The model under review builds one solid part; all positions refer to its coordinate system, in mm. Face numbers are marked on the shaded views. A direction names the side the tool comes from. Give positions to 0.01 mm unless a question says otherwise; leave off trailing zeros. Order: outer loops, then holes, each group sorted by start corner. A loop starts at its lowest first (then second) coordinate and runs counter-clockwise, first axis right, second up. Notation, with made-up numbers: (4, -10) - (22, -10) arc R30 ccw to (22, 25) - close; hole circle Ø1 at (0, 89.25). An arc over 180 degrees is marked (long way). Answer as CSV lines item,"result". Start each with the question number.
from build123d import *

# Parameters (mm, degrees)
SKETCH_1_R          = 18.5
EXTRUDE_1_DEPTH     = 7
EXTRUDE_2_DEPTH     = 4
SKETCH_2_R          = 17.5
CUT_EXTRUDE_1_DEPTH = 3
SKETCH_3_R          = 14
CUT_EXTRUDE_2_DEPTH = 2
CUT_EXTRUDE_5_REACH = 34.299
SKETCH_8_R          = 5.1
CUT_EXTRUDE_6_REACH = 34.16
SKETCH_11_R         = 1.5
FILLET_1_R          = 10
FILLET_2_R          = 5
SKETCH_12_W         = 3
SKETCH_12_H         = 2.288293169
CUT_EXTRUDE_7_DEPTH = 3


with BuildPart() as part:
    # 草图1 → 凸台-拉伸1 (new body)
    with BuildSketch(Plane(origin=(0, 0, 0), x_dir=(0, 0, -1), z_dir=(1, 0, 0))):
        Circle(SKETCH_1_R)
    extrude(amount=EXTRUDE_1_DEPTH)

    # 草图10 → 凸台-拉伸2 (add)
    with BuildSketch(Plane.ZY):
        Polygon((0, 5), (26, 5), (26, -5), (0, -5), (-26, -5), (-26, 5), align=None)
    extrude(amount=-EXTRUDE_2_DEPTH)

    # 草图2 → 切除-拉伸1 (cut)
    with BuildSketch(Plane(origin=(7, 0, 0), x_dir=(0, 0, -1), z_dir=(1, 0, 0))):
        Circle(SKETCH_2_R)
    extrude(amount=-CUT_EXTRUDE_1_DEPTH, mode=Mode.SUBTRACT)

    # 草图3 → 切除-拉伸2 (cut)
    with BuildSketch(Plane(origin=(4, 0, 0), x_dir=(0, 0, -1), z_dir=(1, 0, 0))):
        Circle(SKETCH_3_R)
    extrude(amount=-CUT_EXTRUDE_2_DEPTH, mode=Mode.SUBTRACT)

    # 草图8 → 切除-拉伸5 (cut, up to next)
    with BuildSketch(Plane(origin=(2, 0, 0), x_dir=(0, 0, -1), z_dir=(1, 0, 0)), mode=Mode.PRIVATE) as cut_extrude_5_sk1:
        Circle(SKETCH_8_R)
    cut_extrude_5_tool1 = extrude(cut_extrude_5_sk1.sketch, amount=-CUT_EXTRUDE_5_REACH, mode=Mode.PRIVATE) & part.part
    add(cut_extrude_5_tool1.solids().sort_by_distance((2, 0, 0))[0], mode=Mode.SUBTRACT)

    # 草图11 → 切除-拉伸6 (cut, up to next)
    with BuildSketch(Plane(origin=(4, 0, 0), x_dir=(0, 0, -1), z_dir=(1, 0, 0)), mode=Mode.PRIVATE) as cut_extrude_6_sk1:
        with Locations((-22, 0)):
            Circle(SKETCH_11_R)
    cut_extrude_6_tool1 = extrude(cut_extrude_6_sk1.sketch, amount=-CUT_EXTRUDE_6_REACH, mode=Mode.PRIVATE) & part.part
    # 草图11 → 切除-拉伸6 (cut, up to next)
    with BuildSketch(Plane(origin=(4, 0, 0), x_dir=(0, 0, -1), z_dir=(1, 0, 0)), mode=Mode.PRIVATE) as cut_extrude_6_sk2:
        with Locations((22, 0)):
            Circle(SKETCH_11_R)
    cut_extrude_6_tool2 = extrude(cut_extrude_6_sk2.sketch, amount=-CUT_EXTRUDE_6_REACH, mode=Mode.PRIVATE) & part.part
    add(cut_extrude_6_tool1.solids().sort_by_distance((4, 0, 22))[0], mode=Mode.SUBTRACT)
    add(cut_extrude_6_tool2.solids().sort_by_distance((4, 0, -22))[0], mode=Mode.SUBTRACT)

    # 圆角1
    fillet_1_edges = [part.edges().sort_by_distance(p)[0] for p in [
        (2, 5, -17.811513131),
        (2, 5, 17.811513131),
        (2, -5, 17.811513131),
        (2, -5, -17.811513131),
    ]]
    fillet(fillet_1_edges, radius=FILLET_1_R)

    # 圆角2
    fillet_2_edges = [part.edges().sort_by_distance(p)[0] for p in [
        (2, 5, 26),
        (2, -5, 26),
        (2, -5, -26),
        (2, 5, -26),
    ]]
    fillet(fillet_2_edges, radius=FILLET_2_R)

    # 草图12 → 切除-拉伸7 (cut)
    with BuildSketch(Plane(origin=(7, 0, 0), x_dir=(0, 0, -1), z_dir=(1, 0, 0))):
        with Locations((0, 18.044159171)):
            Rectangle(SKETCH_12_W, SKETCH_12_H)
    extrude(amount=-CUT_EXTRUDE_7_DEPTH, mode=Mode.SUBTRACT)


solid = part.part
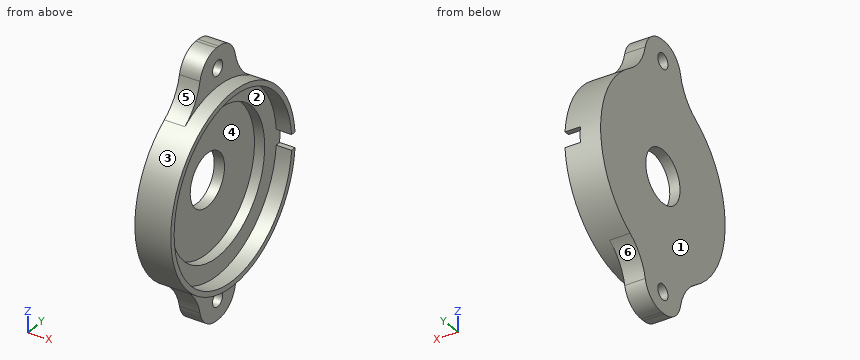
Item 1: For line 1 along Z through (x, y) = (5.1, 0); line 2 along Y through (x, z) = (2.65, 0); line 3 along Y through (x, z) = (3.25, 22), list the stretches that pass through material, from the lowest coordinate up.
Item 2: Machinability: for the marked faces 1 and 2, which of the approach directions +Z, -Z, +X, -X, +Y, -Y give a long, thin tool a straight path to every point of the face, cutting with its end or side? Answer none if there is none.
Item 3: Clearance check with flat-ended pins moving along their axes: pin 1 (4 mm diameter, centred on x = 4, y = -8, fed in from -Z); pin 2 (1.5 mm diameter, centred on y = 14.5, z = 2.5, fed in from +X); pin 3 (4 mm diameter, centred on x = 1, y = 4, fed in from -Z). State where each tip first meets the part, or that it passes through.
Item 4: Take a section at D-D on y = 7.5. Write out the cut boundary in (x, z).
Item 5: Take a section at B-B on x = 3.25. Count the separate pieces of the cut face and the enclosed holes in it, and give its area (3 significant figures).
Item 6: Mouldability with a two-part tool opening along Y and no side actions: class the marked faces 3, 4, 5 and 6 as released by +Y, released by -Y, zero draft, split by the parting line, or undercut.
Item 7: Take a section at A-A on z = 0. Write out the cut boundary in (x, y).
Item 8: Take a section at C-C on y = -9. Write out the cut boundary in (x, z), and give its area (3 significant figures).
Data:
1,line 1,"z = -18.5 to -17.5, 17.5 to 18.5"
1,line 2,"y = -18.5 to -14, 14 to 18.5"
1,line 3,"y = -5.25 to -1.5, 1.5 to 5.25"
2,face 1,"+Z, -Z, -X, +Y, -Y"
2,face 2,"+X"
3,pin 1,"stops at z = -19.87"
3,pin 2,"stops at x = 4"
3,pin 3,"stops at z = -25.72"
4,outline,"(0, -17.62) - (4, -17.62) - (4, -16.91) - (7, -16.91) - (7, -15.81) - (4, -15.81) - (4, -11.82) - (2, -11.82) - (2, 11.82) - (4, 11.82) - (4, 15.81) - (7, 15.81) - (7, 16.91) - (4, 16.91) - (4, 17.62) - (0, 17.62) - close"
5,separate pieces,"1"
5,enclosed holes,"3"
5,area,"609 mm^2"
6,face 3,"split by the parting line"
6,face 4,"undercut"
6,face 5,"released by -Y"
6,face 6,"released by +Y"
7,outline,"(0, -18.5) - (7, -18.5) - (7, -17.5) - (4, -17.5) - (4, -14) - (2, -14) - (2, -5.1) - (0, -5.1) - close; (0, 5.1) - (2, 5.1) - (2, 14) - (4, 14) - (4, 18.5) - (0, 18.5) - close"
8,outline,"(0, -16.23) - (4, -16.23) - (4, -16.16) - (7, -16.16) - (7, -15.01) - (4, -15.01) - (4, -10.72) - (2, -10.72) - (2, 10.72) - (4, 10.72) - (4, 15.01) - (7, 15.01) - (7, 16.16) - (4, 16.16) - (4, 16.23) - (0, 16.23) - close"
8,area,"93.9 mm^2"
